Here's the drawing with two shaded views (mm, measured from the low corner). I have some questions. Coordinates: 2 decimals unless noted, no trailing zeros. Order: outer loops, then holes, each group sorted by start corner. A loop starts at its lowest first (then second) coordinate and runs counter-clockwise, first axis right, second up. Notation, with made-up numbers: (73, 4.25) -> (102, 4.25) arc R27 cw to (102, 35.25) -> close; hole circle Ø6 at (-11, 82.5). An arc over 180 degrees is marked (long way). Return JSON: item names as keys, results as strings. Group by question number.
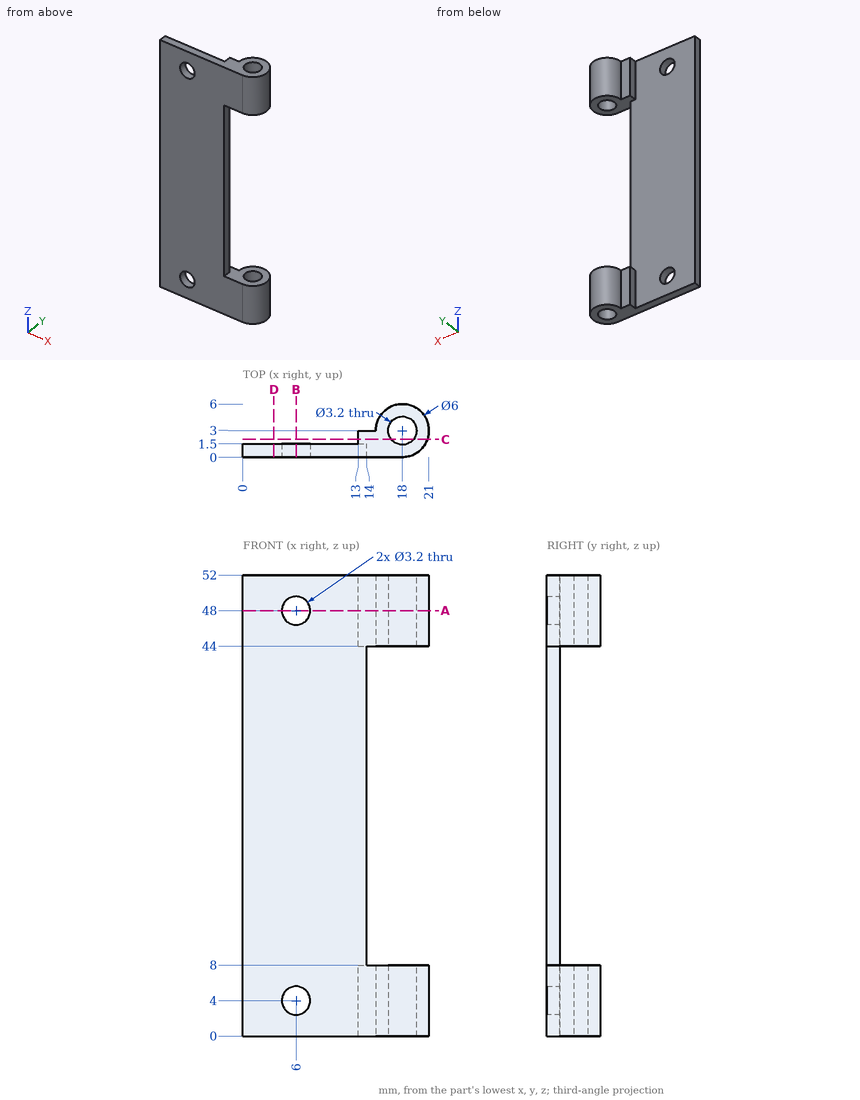
Q1. I want a section at D-D on x = 3.5. Please give me the cut outline in (y, z).
Q2. I need wall thicknesses on line 1 along Z through (x, y) = (6, 0.45); line 2 along Y through (x, z) = (18, 1.5); line 3 along X through (y, z) = (3.15, 49). Which ranges of each line are inside material? Lowest first, please. Write a range as from..to.
Q3. I want a section at A-A on z = 48. Please give me the cut outline in (x, y).
Q4. I want a section at B-B on x = 6. Please give me the cut outline in (y, z).
Q5. I want a section at C-C on y = 2. Please give me the cut outline in (x, z).
Q6. I'm going to push flat-ended pins straight in: pin 1 Ø3 at (y, z) = (1, 21) entering from +X; pin 2 Ø11 at (x, z) = (7.5, 16) entering from +Y; pin 3 Ø1.9 at (x, y) = (18, 3) entering from -Z. Where does each tip first touch, or does it pass through?
Response values:
{
 "1": {"outline": "(0, 0) -> (1.5, 0) -> (1.5, 52) -> (0, 52) -> close"},
 "2": {"line 1": "z = 0..2.4, 5.6..46.4, 49.6..52", "line 2": "y = 0..1.4, 4.6..6", "line 3": "x = 15..16.41, 19.59..21"},
 "3": {"outline": "(0, 0) -> (4.4, 0) -> (4.4, 1.5) -> (0, 1.5) -> close; (7.6, 0) -> (18, 0) arc R3 ccw (long way) to (15, 3) -> (13, 3) -> (13, 1.5) -> (7.6, 1.5) -> close; hole circle Ø3.2 at (18, 3)"},
 "4": {"outline": "(0, 0) -> (1.5, 0) -> (1.5, 2.4) -> (0, 2.4) -> close; (0, 5.6) -> (1.5, 5.6) -> (1.5, 46.4) -> (0, 46.4) -> close; (0, 49.6) -> (1.5, 49.6) -> (1.5, 52) -> (0, 52) -> close"},
 "5": {"outline": "(13, 0) -> (16.75, 0) -> (16.75, 8) -> (13, 8) -> close; (13, 44) -> (16.75, 44) -> (16.75, 52) -> (13, 52) -> close; (19.25, 0) -> (20.83, 0) -> (20.83, 8) -> (19.25, 8) -> close; (19.25, 44) -> (20.83, 44) -> (20.83, 52) -> (19.25, 52) -> close"},
 "6": {"pin 1": "stops at x = 14", "pin 2": "stops at y = 1.5", "pin 3": "passes through"}
}
